```python
from build123d import *

# Parameters (mm, degrees)
F0_W     = 48.26
F0_H     = 38.1
F1_DEPTH = 15.24
F3_T     = -0.254
F4_D     = 6.858
F6_D     = 5.08


with BuildPart() as f1:
    # F0 (on Front) → F1 (new body)
    with BuildSketch(Plane.XZ):
        Rectangle(F0_W, F0_H)
    extrude(amount=F1_DEPTH)

    # F3
    f3_openings = [f1.faces().sort_by_distance(p)[0] for p in [
        (0, 0, 0),
        (24.13, -7.62, 0),
    ]]
    offset(amount=F3_T, openings=f3_openings)

    # F4 (through all)
    with Locations(Plane.XZ.offset(15.24)):
        with Locations((-16.383, 0)):
            Hole(F4_D / 2)

    # F6 (through all)
    with Locations(Plane.XZ.offset(15.24)):
        with Locations((0, 0)):
            Hole(F6_D / 2)


solid = f1.part
```
For this review, take the finished solid that the model builds, in its own axes (mm). A direction names the side the tool comes from. Coordinates: 2 decimals unless noted, no trailing zeros. Loops run counter-clockwise (first coordinate to the right, second up) from the corner with the lowest first, then second, coordinate; pieces in that order, holes last.
1. For line 1 (Z direction, x = -17, y = -9.5); line 2 (Z direction, x = 0, y = -15.1); line 3 (Y direction, x = 11, z = -3.5), list the stretches that pass through material, from the lowest coordinate up.
2. Add section A-A, the plane x = 0. Give the boundary of the cut face in (y, z).
3. Add section B-B, the plane z = 0. Give the boundary of the cut face in (x, y).
4. Add section D-D, the plane y = -5.75. Give the boundary of the cut face in (x, z).
5. For faces 1 (the flat face through (0, -14.986, 4)), 2 (the flat face through (0, -8, 19.05)), list the 3-axis set-ups (+Z, -Z, +X, -X, +Y, -Y) from which the entire face can be reached by the end or side of a thin tool; tool diameter is ignored.
6. Insertion check: P1, Ø4, axis at x = 0, z = 0, coming from the -Y side (3 decimals); P2, Ø4, axis at y = -2, z = 9.5, coming from the +X side; P3, Ø8, axis at x = -15.5, z = 14.5, coming from the +Y side. Each pin has a flat end and moves straight along its axis. Give the tip position at first contact, or say it passes through.
7. Add section C-C, the plane x = 12.5. Give the boundary of the cut face in (y, z).
Result:
1. line 1: z = -19.05 to -18.8, 18.8 to 19.05
1. line 2: z = -19.05 to -2.54, 2.54 to 19.05
1. line 3: y = -15.24 to -14.99
2. outline: (-15.24, -19.05) - (0, -19.05) - (0, -18.8) - (-14.99, -18.8) - (-14.99, -2.54) - (-15.24, -2.54) - close; (-15.24, 2.54) - (-14.99, 2.54) - (-14.99, 18.8) - (0, 18.8) - (0, 19.05) - (-15.24, 19.05) - close
3. outline: (-24.13, -15.24) - (-19.81, -15.24) - (-19.81, -14.99) - (-23.88, -14.99) - (-23.88, 0) - (-24.13, 0) - close; (-12.95, -15.24) - (-2.54, -15.24) - (-2.54, -14.99) - (-12.95, -14.99) - close; (2.54, -15.24) - (24.13, -15.24) - (24.13, -14.99) - (2.54, -14.99) - close
4. outline: (-24.13, -19.05) - (24.13, -19.05) - (24.13, -18.8) - (-23.88, -18.8) - (-23.88, 18.8) - (24.13, 18.8) - (24.13, 19.05) - (-24.13, 19.05) - close
5. face 1: +X, +Y
5. face 2: +Z, +X, -X, +Y, -Y
6. P1: passes through
6. P2: stops at x = -23.88
6. P3: stops at y = -14.99
7. outline: (-15.24, -19.05) - (0, -19.05) - (0, -18.8) - (-14.99, -18.8) - (-14.99, 18.8) - (0, 18.8) - (0, 19.05) - (-15.24, 19.05) - close
